```python
from build123d import *

# Parameters (mm, degrees)
SKETCH1_W           = 609.6
SKETCH1_H           = 355.6
BOSS_EXTRUDE1_DEPTH = 15.24
SKETCH2_R           = 15.24
CUT_EXTRUDE1_DEPTH  = 3.81
SKETCH3_W           = 584.2
SKETCH3_H           = 330.2
BOSS_EXTRUDE2_DEPTH = 330.2
SKETCH4_W           = 172.72
SKETCH4_H           = 314.96
SKETCH4_W_2         = 365.76
CUT_EXTRUDE2_DEPTH  = 330.2
SKETCH6_W           = 15.24
SKETCH6_H           = 314.96
CUT_EXTRUDE4_DEPTH  = 12.7
SKETCH8_W           = 584.2
SKETCH8_H           = 330.2
BOSS_EXTRUDE4_DEPTH = 12.7
SKETCH11_R          = 3.81
CUT_EXTRUDE5_DEPTH  = 5.08
SKETCH12_R          = 3.81
CUT_EXTRUDE6_DEPTH  = 5.08
SKETCH13_R          = 5.08
CUT_EXTRUDE7_DEPTH  = 12.7


with BuildPart() as part:
    # Sketch1 → Boss-Extrude1 (new body)
    with BuildSketch(Plane(origin=(0, 0, 0), x_dir=(1, 0, 0), z_dir=(0, 1, 0))):
        with Locations((304.8, 177.8)):
            Rectangle(SKETCH1_W, SKETCH1_H)
    extrude(amount=BOSS_EXTRUDE1_DEPTH)

    # Sketch2 → Cut-Extrude1 (cut)
    with BuildSketch(Plane(origin=(0, 0, 0), x_dir=(-1, 0, 0), z_dir=(0, -1, 0))):
        with Locations((-558.8, 50.8)):
            Circle(SKETCH2_R)
        with Locations((-558.8, 304.8)):
            Circle(SKETCH2_R)
        with Locations((-50.8, 50.8)):
            Circle(SKETCH2_R)
        with Locations((-50.8, 304.8)):
            Circle(SKETCH2_R)
    extrude(amount=-CUT_EXTRUDE1_DEPTH, mode=Mode.SUBTRACT)

    # Sketch3 → Boss-Extrude2 (add)
    with BuildSketch(Plane(origin=(0, 15.24, 0), x_dir=(1, 0, 0), z_dir=(0, 1, 0))):
        with Locations((304.8, 177.8)):
            Rectangle(SKETCH3_W, SKETCH3_H)
    extrude(amount=BOSS_EXTRUDE2_DEPTH)

    # Sketch4 → Cut-Extrude2 (cut)
    with BuildSketch(Plane.XY.offset(-12.7)):
        with Locations((495.3, 172.72)):
            Rectangle(SKETCH4_W, SKETCH4_H)
        with Locations((210.82, 172.72)):
            Rectangle(SKETCH4_W_2, SKETCH4_H)
    extrude(amount=-CUT_EXTRUDE2_DEPTH, mode=Mode.SUBTRACT)

    # Sketch6 → Cut-Extrude4 (cut)
    with BuildSketch(Plane.XY.offset(-12.7)):
        with Locations((401.32, 172.72)):
            Rectangle(SKETCH6_W, SKETCH6_H)
    extrude(amount=-CUT_EXTRUDE4_DEPTH, mode=Mode.SUBTRACT)

    # Sketch8 → Boss-Extrude4 (add)
    with BuildSketch(Plane(origin=(0, 0, -342.9), x_dir=(-1, 0, 0), z_dir=(0, 0, -1))):
        with Locations((-304.8, 180.34)):
            Rectangle(SKETCH8_W, SKETCH8_H)
    extrude(amount=-BOSS_EXTRUDE4_DEPTH)

    # Sketch11 → Cut-Extrude5 (cut)
    with BuildSketch(Plane(origin=(0, 15.24, 0), x_dir=(1, 0, 0), z_dir=(0, 1, 0))):
        with Locations((575.31, 20.32)):
            Circle(SKETCH11_R)
    extrude(amount=-CUT_EXTRUDE5_DEPTH, mode=Mode.SUBTRACT)

    # Sketch12 → Cut-Extrude6 (cut)
    with BuildSketch(Plane(origin=(0, 330.2, 0), x_dir=(-1, 0, 0), z_dir=(0, -1, 0))):
        with Locations((-575.31, 20.32)):
            Circle(SKETCH12_R)
    extrude(amount=-CUT_EXTRUDE6_DEPTH, mode=Mode.SUBTRACT)

    # Sketch13 → Cut-Extrude7 (cut)
    with BuildSketch(Plane(origin=(0, 345.44, 0), x_dir=(-1, 0, 0), z_dir=(0, 1, 0))):
        with Locations((-546.1, -63.5)):
            Circle(SKETCH13_R)
        with Locations((-63.5, -63.5)):
            Circle(SKETCH13_R)
        with Locations((-63.5, -292.1)):
            Circle(SKETCH13_R)
        with Locations((-546.1, -292.1)):
            Circle(SKETCH13_R)
    extrude(amount=-CUT_EXTRUDE7_DEPTH, mode=Mode.SUBTRACT)


solid = part.part
```
Here's how the part is built. I have some questions about the finished solid (model axes, mm). A direction names the side the tool comes from. Give positions to 0.01 mm unless a question says otherwise; leave off trailing zeros. Write each loop counter-clockwise with the first axis right and the second up, starting at its lowest first coordinate (ties: lowest second). Pieces come first, ordered by that corner, then holes.
(1) Will these pins go through, and if not, where does the flat tip stop? pin 1 (1 mm diameter, centred on y = 140, z = -85.5, fed in from +X); pin 2 (2 mm diameter, centred on x = 307.5, y = 41.5, fed in from -Z); pin 3 (1.5 mm diameter, centred on x = 161.5, y = 86, fed in from +Z).
Output values:
pin 1: stops at x = 596.9
pin 2: stops at z = -342.9
pin 3: stops at z = -330.2
(2) Imagine slicing it at B-B, the plane x = 365. Write out the boundary of the cut face in (y, z), and give its area (3 significant figures).
Output values:
outline: (0, -355.6) - (15.24, -355.6) - (15.24, -342.9) - (345.44, -342.9) - (345.44, -12.7) - (330.2, -12.7) - (330.2, -330.2) - (15.24, -330.2) - (15.24, 0) - (0, 0) - close
area: 14,500 mm2
(3) Imagine slicing it at C-C, the plane y = 154.5. Write out the boundary of the cut face in (x, z), and give its area (3 significant figures).
Output values:
outline: (12.7, -342.9) - (596.9, -342.9) - (596.9, -12.7) - (581.66, -12.7) - (581.66, -330.2) - (408.94, -330.2) - (408.94, -25.4) - (393.7, -25.4) - (393.7, -330.2) - (27.94, -330.2) - (27.94, -12.7) - (12.7, -12.7) - close
area: 21,700 mm2
(4) On a 3-axis mill with a long thin cutter (end or side, diameter ignored), from which of +Z, -Z, +X, -X, +Y, -Y can I reach the whole of each face in a straight line? I mean faces 4 (the face through (213, 175, -330.2)), 5 (the face through (301, 178, -342.9)), 6 (the face through (559, 3.81, -51)). Say none if no direction works.
Output values:
face 4: +Z
face 5: -Z, +X, -X, +Y
face 6: -Y
(5) Imagine slicing it at A-A, the plane z = -245. Write out the boundary of the cut face in (x, y), and give its area (3 significant figures).
Output values:
outline: (0, 0) - (609.6, 0) - (609.6, 15.24) - (596.9, 15.24) - (596.9, 345.44) - (12.7, 345.44) - (12.7, 15.24) - (0, 15.24) - close; hole (27.94, 15.24) - (393.7, 15.24) - (393.7, 330.2) - (27.94, 330.2) - close; hole (408.94, 15.24) - (581.66, 15.24) - (581.66, 330.2) - (408.94, 330.2) - close
area: 32,600 mm2
(6) Thinking about a two-plate mould opening in Y: for faces 1 (the face through (301, 330.2, -169)), 2 (the face through (609.6, 8, -175)), 3 (the face through (51, 3.81, -51)), which applies, pulls with the +Y half, pulls with the -Y half, needs draft (parallel to the pull), parting line crosses it, or undercut?
Output values:
face 1: undercut
face 2: needs draft
face 3: pulls with the -Y half
(7) Imagine slicing it at D-D, the plane z = -304.8. Write out the boundary of the cut face in (x, y), and give its area (3 significant figures).
Output values:
outline: (0, 0) - (35.56, 0) - (35.56, 3.81) - (66.04, 3.81) - (66.04, 0) - (543.56, 0) - (543.56, 3.81) - (574.04, 3.81) - (574.04, 0) - (609.6, 0) - (609.6, 15.24) - (596.9, 15.24) - (596.9, 345.44) - (12.7, 345.44) - (12.7, 15.24) - (0, 15.24) - close; hole (27.94, 15.24) - (393.7, 15.24) - (393.7, 330.2) - (27.94, 330.2) - close; hole (408.94, 15.24) - (581.66, 15.24) - (581.66, 330.2) - (408.94, 330.2) - close
area: 32,400 mm2
(8) If I drill on L1, parallel to X at y = 337, z = -63; L2, parallel to Z at x = 546.1, y = 340.5; L3, parallel to Z at x = 50, y = 1, over which ranges is the centre line in solid material (lowest first)?
Output values:
L1: x = 12.7 to 58.44, 68.56 to 541.04, 551.16 to 596.9
L2: z = -342.9 to -297.18, -287.02 to -68.58, -58.42 to -12.7
L3: z = -355.6 to -320.02, -289.58 to -66.02, -35.58 to 0
